from build123d import *

# Parameters (mm, degrees)
EXTRUDE_2_DEPTH      = 8
EXTRUDE_2_DEPTH_BACK = 8
SKETCH_1_W           = 20.1
SKETCH_1_H           = 9
SKETCH_1_R           = 1.4
SKETCH_1_4_W         = 20.1
SKETCH_1_4_H         = 3
EXTRUDE_3_DEPTH      = 28
SKETCH_3_R           = 0.7
CUT_EXTRUDE_1_DEPTH  = 28


with BuildPart() as part:
    # Sketch 1 → Extrude 2 (new, two sides: drawn at the far end of the back side and taken through both)
    # profile 1 of 5: a face of its own
    with BuildSketch(Plane(origin=(0, 0, 0), x_dir=(1, 0, 0), z_dir=(0, 1, 0)).offset(-EXTRUDE_2_DEPTH_BACK)):
        with Locations((-26.1, -24.85)):
            Rectangle(SKETCH_1_W, SKETCH_1_H)
        with Locations(Location((-21.075, -24.125, 0), (0, 0, 270))):
            Circle(SKETCH_1_R, mode=Mode.SUBTRACT)
        with Locations(Location((-31.125, -24.125, 0), (0, 0, 270))):
            Circle(SKETCH_1_R, mode=Mode.SUBTRACT)
    # profile 2 of 5: a face of its own
    with BuildSketch(Plane(origin=(0, 0, 0), x_dir=(1, 0, 0), z_dir=(0, 1, 0)).offset(-EXTRUDE_2_DEPTH_BACK)):
        Polygon((-16.05, 29.35), (-10.05, 29.35), (-10.05, 20.35), (-10.05, -20.35), (-10.05, -29.35), (-16.05, -29.35), (-16.05, -20.35), (-16.05, 20.35), align=None)
    # profile 3 of 5: a face of its own
    with BuildSketch(Plane(origin=(0, 0, 0), x_dir=(1, 0, 0), z_dir=(0, 1, 0)).offset(-EXTRUDE_2_DEPTH_BACK)):
        with Locations((0, -24.85)):
            Rectangle(SKETCH_1_W, SKETCH_1_H)
        with Locations(Location((5.025, -24.125, 0), (0, 0, 270))):
            Circle(SKETCH_1_R, mode=Mode.SUBTRACT)
        with Locations(Location((-5.025, -24.125, 0), (0, 0, 270))):
            Circle(SKETCH_1_R, mode=Mode.SUBTRACT)
    # profile 4 of 5: a face of its own
    with BuildSketch(Plane(origin=(0, 0, 0), x_dir=(1, 0, 0), z_dir=(0, 1, 0)).offset(-EXTRUDE_2_DEPTH_BACK)):
        with Locations((0, 24.85)):
            Rectangle(SKETCH_1_W, SKETCH_1_H)
        with Locations(Location((-5.025, 24.125, 0), (0, 0, 270))):
            Circle(SKETCH_1_R, mode=Mode.SUBTRACT)
        with Locations(Location((5.025, 24.125, 0), (0, 0, 270))):
            Circle(SKETCH_1_R, mode=Mode.SUBTRACT)
    # profile 5 of 5: a face of its own
    with BuildSketch(Plane(origin=(0, 0, 0), x_dir=(1, 0, 0), z_dir=(0, 1, 0)).offset(-EXTRUDE_2_DEPTH_BACK)):
        with Locations((-26.1, 24.85)):
            Rectangle(SKETCH_1_W, SKETCH_1_H)
        with Locations(Location((-31.125, 24.125, 0), (0, 0, 270))):
            Circle(SKETCH_1_R, mode=Mode.SUBTRACT)
        with Locations(Location((-21.075, 24.125, 0), (0, 0, 270))):
            Circle(SKETCH_1_R, mode=Mode.SUBTRACT)
    extrude(amount=EXTRUDE_2_DEPTH + EXTRUDE_2_DEPTH_BACK)

    # Sketch 1_4 → Extrude 3 (add)
    with BuildSketch(Plane(origin=(0, 0, 0), x_dir=(1, 0, 0), z_dir=(0, 1, 0))):
        with Locations((0, -30.85)):
            Rectangle(SKETCH_1_4_W, SKETCH_1_4_H)
    extrude(amount=EXTRUDE_3_DEPTH)

    # Sketch 3 → Cut-Extrude 1 (cut)
    with BuildSketch(Plane(origin=(0, 0, 29.35), x_dir=(-1, 0, 0), z_dir=(0, 0, -1))):
        with Locations((-2.5, 23)):
            Circle(SKETCH_3_R)
        with Locations((2.5, 23)):
            Circle(SKETCH_3_R)
    extrude(amount=-CUT_EXTRUDE_1_DEPTH, mode=Mode.SUBTRACT)


solid = part.part
The model under review builds one solid part; all positions refer to its coordinate system, in mm. A direction names the side the tool comes from. Give positions to 0.01 mm unless a question says otherwise; leave off trailing zeros. Loops run counter-clockwise (first coordinate to the right, second up) from the corner with the lowest first, then second, coordinate; pieces in that order, holes last. Notation, with made-up numbers: (42, 3.5) -> (85, 3.5) arc R19 cw to (85, 37.5) -> close; hole circle Ø5 at (60.5, 55). An arc over 180 degrees is marked (long way). Answer as a JSON object with one key per item and string values. Group by question number.
Q1. Take a section at A-A (x = -25.5). Write out the cut boundary in (y, z), plus the area to 3 significant figures.
Q2. Take a section at C-C (x = -2.5). Write out the cut boundary in (y, z).
Q3. Wall thickness on line 1 along Y through (x, z) = (2.5, 30.45); line 2 along X through (y, z) = (-3, 24); line 3 along Z through (x, y) = (6, 1): over which ranges is each line inside the solid? List them lowest first.
Q4. Insertion check: pin 1 (1.5 mm diameter, centred on x = -17.5, z = 5, fed in from -Y) (3 decimals); pin 2 (2 mm diameter, centred on x = -29, y = -1, fed in from +Z); pin 3 (5 mm diameter, centred on y = 0.5, z = 8, fed in from +X); pin 4 (3 mm diameter, centred on x = -21.075, z = 24.125, fed in from +Y). Each pin has a flat end and moves straight along its axis. Give the tip position at first contact, or say it passes through.
Q5. Take a section at B-B (y = 23). Write out the cut boundary in (x, z), plus the area to 3 significant figures.
Q6. Draft analysis for pull direction X (two halves, no side actions). For faces 5 (the cylindrical face through (-29.945, -0.112, 24.878)), 6 (the flat face through (-10.05, 14, 31)), 7 (the flat face through (0, 14, 32.35)), state which applies: pulls with the +X half, pulls with the -X half, needs draft (parallel to the pull), parting line crosses it, or undercut.
Q7. Take a section at D-D (z = 24). Write out the cut boundary in (x, y).
Q8. Tool access review of faces 1 (the flat face through (0, 0, 31)), 2 (the flat face through (0, 18, 29.35)), 3 (the flat face through (-26, 0, -20.35)), 4 (the flat face through (0, 0, -20.35)): name each direction out of +Z, -Z, +X, -X, +Y, -Y from which nothing blocks a thin tool from reaching the whole face with its end or side.
Answer below:
{
 "1": {"outline": "(-8, -29.35) -> (8, -29.35) -> (8, -20.35) -> (-8, -20.35) -> close; (-8, 20.35) -> (8, 20.35) -> (8, 29.35) -> (-8, 29.35) -> close", "area": "288 mm2"},
 "2": {"outline": "(-8, -29.35) -> (8, -29.35) -> (8, -20.35) -> (-8, -20.35) -> close; (-8, 20.35) -> (8, 20.35) -> (8, 29.35) -> (22.3, 29.35) -> (22.3, 32.35) -> (0, 32.35) -> (0, 29.35) -> (-8, 29.35) -> close; (23.7, 29.35) -> (28, 29.35) -> (28, 32.35) -> (23.7, 32.35) -> close"},
 "3": {"line 1": "y = 0 to 22.3, 23.7 to 28", "line 2": "x = -36.15 to -32.52, -29.73 to -22.47, -19.68 to -6.42, -3.63 to 3.63, 6.42 to 10.05", "line 3": "z = -29.35 to -25.13, -23.12 to -20.35, 20.35 to 23.12, 25.13 to 32.35"},
 "4": {"pin 1": "passes through", "pin 2": "stops at z = 29.35", "pin 3": "stops at x = -10.05", "pin 4": "stops at y = 8"},
 "5": {"outline": "(-10.05, 29.35) -> (-3.2, 29.35) -> (-3.2, 32.35) -> (-10.05, 32.35) -> close; (-1.8, 29.35) -> (1.8, 29.35) -> (1.8, 32.35) -> (-1.8, 32.35) -> close; (3.2, 29.35) -> (10.05, 29.35) -> (10.05, 32.35) -> (3.2, 32.35) -> close", "area": "51.9 mm2"},
 "6": {"face 5": "undercut", "face 6": "pulls with the -X half", "face 7": "needs draft"},
 "7": {"outline": "(-36.15, -8) -> (-32.52, -8) -> (-32.52, 8) -> (-36.15, 8) -> close; (-29.73, -8) -> (-22.47, -8) -> (-22.47, 8) -> (-29.73, 8) -> close; (-19.68, -8) -> (-6.42, -8) -> (-6.42, 8) -> (-19.68, 8) -> close; (-3.63, -8) -> (3.63, -8) -> (3.63, 8) -> (-3.63, 8) -> close; (6.42, -8) -> (10.05, -8) -> (10.05, 8) -> (6.42, 8) -> close"},
 "8": {"face 1": "+Z, +X, -X, -Y", "face 2": "-Z, +X, -X, +Y", "face 3": "-X, +Y, -Y", "face 4": "+X, +Y, -Y"}
}
